The listing builds one solid part. Answer for the finished solid, in the listing's coordinates (mm). Face numbers are marked on the shaded views. A direction names the side the tool comes from. Coordinates: 2 decimals unless noted, no trailing zeros. Write each loop counter-clockwise with the first axis right and the second up, starting at its lowest first coordinate (ties: lowest second). Pieces come first, ordered by that corner, then holes.
(1) The part is cut by section A-A on y = 6. Determine the outline of the cut face in (x, z).
(2) The part is cut by section D-D on z = -4.5. Determine the outline of the cut face in (x, y).
(3) For a pull along Z with two mould halves and no side action, classify the marked faces 4, 5, 6 and 7 as +Z half, -Z half, draft (parallel to the pull), parting line (faces both ways), or undercut.
(4) Which of the six approach directions +Z, -Z, +X, -X, +Y, -Y give full straight-line access (tool end or side, diameter ignored) to the marked faces 1, 2 and 3?
(5) Given P1, Ø1, axis at x = 0.5, z = 0, coming from the -Y side; P2, Ø0.9, axis at x = 0.5, y = 10.5, coming from the -Z side, each flat-ended and moving along its own axis, determine where each tip first touches the part or whether it passes through.
(6) Straight lines are drawn through the part: line 1 (Y direction, x = 0.15, z = -0.25); line 2 (Z direction, x = 0.6, y = 1.25); line 3 (Z direction, x = 0.15, y = 1). For each, find the intervals that lie inside material, in ascending order.
(7) The part is cut by section B-B on x = 0.65. Determine the outline of the cut face in (y, z).
(8) The part is cut by section C-C on z = 3.25. Determine the outline of the cut face in (x, y).
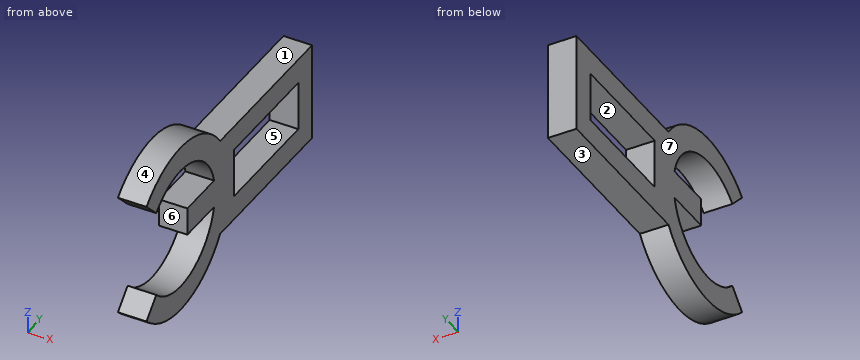
from build123d import *

# Parameters (mm, degrees)
SKETCH1_W           = 6
SKETCH1_H           = 10
SKETCH1_W_2         = 3
SKETCH1_H_2         = 7
SKETCH1_W_3         = 1.7
SKETCH1_H_3         = 3
BOSS_EXTRUDE1_DEPTH = 1.7272


with BuildPart() as part:
    # Sketch1 → Boss-Extrude1 (new body)
    # profile 1 of 3: a face of its own
    with BuildSketch(Plane(origin=(0, 0, 0), x_dir=(0, 0, -1), z_dir=(1, 0, 0))):
        with BuildLine():
            Line((-2.644579362, -2.644579362), (-3.705239533, -3.705239533))
            ThreePointArc((-3.705239533, -3.705239533), (-4.84112875, 2.005261186), (0, 5.24))
            ThreePointArc((0, 5.24), (4.84112875, 2.005261186), (3.705239533, -3.705239533))
            Line((3.705239533, -3.705239533), (2.644579362, -2.644579362))
            ThreePointArc((2.644579362, -2.644579362), (0, 3.74), (-2.644579362, -2.644579362))
        make_face()
    # profile 2 of 3: a face of its own
    with BuildSketch(Plane(origin=(0, 0, 0), x_dir=(0, 0, -1), z_dir=(1, 0, 0))):
        with Locations((0, 9.296230906)):
            Rectangle(SKETCH1_W, SKETCH1_H)
        with Locations((0, 9.296230906)):
            Rectangle(SKETCH1_W_2, SKETCH1_H_2, mode=Mode.SUBTRACT)
    # profile 3 of 3: a face of its own
    with BuildSketch(Plane(origin=(0, 0, 0), x_dir=(0, 0, -1), z_dir=(1, 0, 0))):
        with Locations((0, 2.24)):
            Rectangle(SKETCH1_W_3, SKETCH1_H_3)
    extrude(amount=BOSS_EXTRUDE1_DEPTH)


solid = part.part
Model answer:
1. outline: (0, -3) - (1.73, -3) - (1.73, -1.5) - (0, -1.5) - close; (0, 1.5) - (1.73, 1.5) - (1.73, 3) - (0, 3) - close
2. outline: (0, -2.68) - (1.73, -2.68) - (1.73, 2.68) - (0, 2.68) - close
3. face 4: +Z half
3. face 5: undercut
3. face 6: undercut
3. face 7: draft
4. face 1: +Z, +X, -X, +Y
4. face 2: +X, -X
4. face 3: -Z, +X, -X, +Y
5. P1: stops at y = 0.74
5. P2: stops at z = -3
6. line 1: y = 0.74 to 5.8, 12.8 to 14.3
6. line 2: z = -5.09 to -3.52, -0.85 to 0.85, 3.52 to 5.09
6. line 3: z = -5.14 to -3.6, -0.85 to 0.85, 3.6 to 5.14
7. outline: (-3.71, -3.71) arc R5.24 ccw to (4.3, -3) - (14.3, -3) - (14.3, 3) - (4.3, 3) arc R5.24 ccw to (-3.71, 3.71) - (-2.64, 2.64) arc R3.74 cw to (3.64, 0.85) - (0.74, 0.85) - (0.74, -0.85) - (3.64, -0.85) arc R3.74 cw to (-2.64, -2.64) - close; hole (5.8, -1.5) - (12.8, -1.5) - (12.8, 1.5) - (5.8, 1.5) - close
8. outline: (0, -3.25) - (1.73, -3.25) - (1.73, -1.85) - (0, -1.85) - close; (0, 1.85) - (1.73, 1.85) - (1.73, 4.11) - (0, 4.11) - close
